Answer from the drawing. Dimensions are ordinates in mm from the lowest x, y and z of the part. A direction names the side the tool comes from. Give positions to 0.01 mm unless a question says otherwise; leave off trailing zeros. Order: outer loops, then holes, each group sorted by start corner. A loop starts at its lowest first (then second) coordinate and runs counter-clockwise, first axis right, second up. Notation, with made-up numbers: (-13, 11.5) - (19, 11.5) arc R24 cw to (19, 30.5) - close; hole circle Ø10 at (87.5, 66). An arc over 180 degrees is marked (long way). Write each question's results on one line, items separated by ' | '.
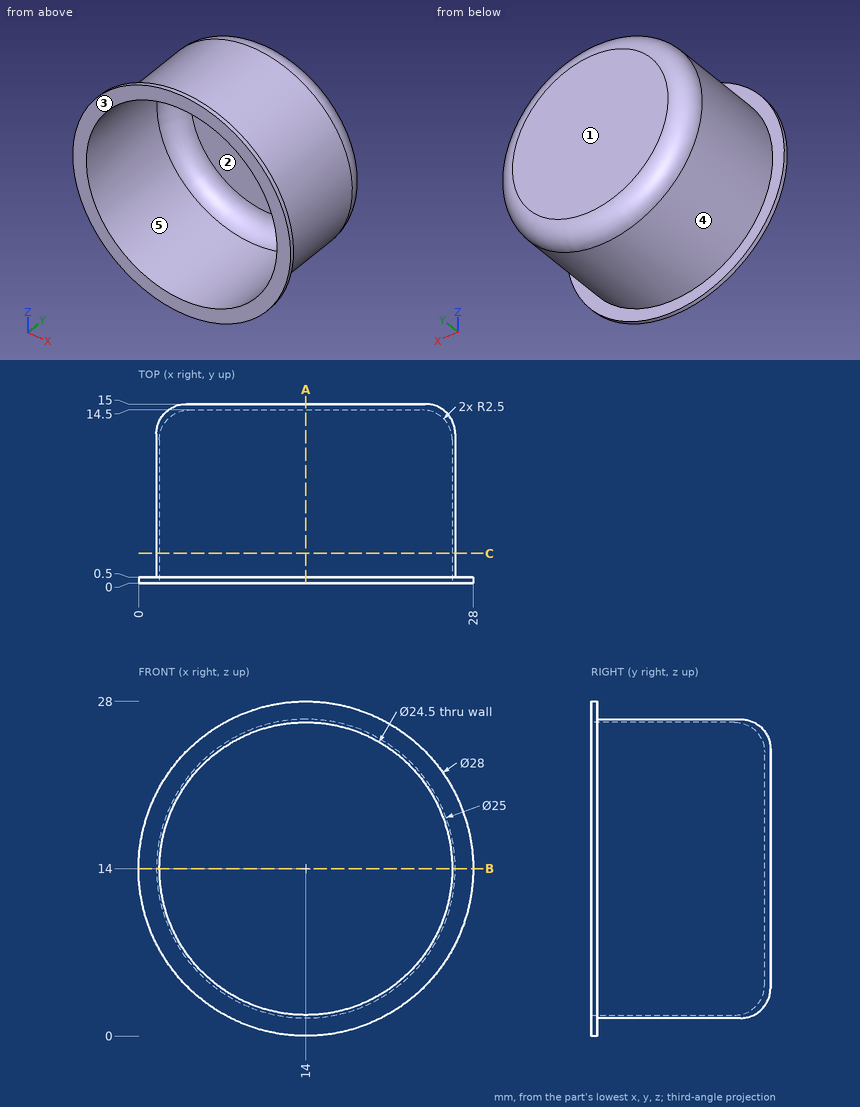
1. A cutting plane is placed at A-A, the plane x = 14. Write down the section's boundary in (y, z).
Answer list:
outline: (0, 0) - (0.5, 0) - (0.5, 1.5) - (12.5, 1.5) arc R2.5 ccw to (15, 4) - (15, 24) arc R2.5 ccw to (12.5, 26.5) - (0.5, 26.5) - (0.5, 28) - (0, 28) - (0, 26.25) - (12, 26.25) arc R2.5 cw to (14.5, 23.75) - (14.5, 4.25) arc R2.5 cw to (12, 1.75) - (0, 1.75) - close
2. A tool of negligible diameter and unlimited length cuts with its end or side. For the marked faces 1 and 2, from which of +Z, -Z, +X, -X, +Y, -Y can it reach the whole face along a straight path? Write none if from no direction.
Answer list:
face 1: +Z, -Z, +X, -X, +Y | face 2: -Y
3. A cutting plane is placed at C-C, the plane y = 2.5. Write down the section's boundary in (x, z).
Answer list:
outline: circle Ø25 at (14, 14); hole circle Ø24.5 at (14, 14)
4. Given P1, Ø8, axis at x = 25, y = 6.5, coming from the +Z side; P2, Ø12, axis at x = 18, z = 16.5, coming from the -Y side; P3, Ø10, axis at x = 19.5, z = 4, coming from the -Y side; P4, Ø1, axis at x = 5.5, y = 3.5, coming from the -Z side, each flat-ended and moving along its own axis, determine where each tip first touches the part or whether it passes through.
Answer list:
P1: z = 24.36 | P2: y = 14.31 | P3: y = 0 | P4: z = 4.4
5. Determine the mould class of the marked faces 3, 4 and 5 for opening direction X: +X half, -X half, draft (parallel to the pull), parting line (faces both ways), or undercut.
Answer list:
face 3: draft | face 4: parting line | face 5: undercut
6. A cutting plane is placed at B-B, the plane z = 14. Write down the section's boundary in (x, y).
Answer list:
outline: (0, 0) - (1.75, 0) - (1.75, 12) arc R2.5 cw to (4.25, 14.5) - (23.75, 14.5) arc R2.5 cw to (26.25, 12) - (26.25, 0) - (28, 0) - (28, 0.5) - (26.5, 0.5) - (26.5, 12.5) arc R2.5 ccw to (24, 15) - (4, 15) arc R2.5 ccw to (1.5, 12.5) - (1.5, 0.5) - (0, 0.5) - close
7. Straight lines are drawn through the part: line 1 (X direction, y = 3, z = 14); line 2 (Y direction, x = 26, z = 8); line 3 (X direction, y = 9.5, z = 4.75). For each, find the intervals that lie inside material, in ascending order. Write a range as [from, to].
Answer list:
line 1: [1.5, 1.75], [26.25, 26.5] | line 2: [0, 0.5] | line 3: [5.59, 5.97], [22.03, 22.41]
